Here's how the part is built. I have some questions about the finished solid (model axes, mm). A direction names the side the tool comes from. Coordinates: 2 decimals unless noted, no trailing zeros. Write each loop counter-clockwise with the first axis right and the second up, starting at its lowest first coordinate (ties: lowest second). Pieces come first, ordered by that corner, then holes.
from build123d import *

# Parameters (mm, degrees)
F3_DEPTH = 1.3
F4_R     = 2
F5_DEPTH = 25
F6_SIZE  = 0.3


with BuildPart() as f1:
    # F0 (on Front) → F1 (revolve)
    with BuildSketch(Plane.XZ):
        with BuildLine():
            Line((-3.8, 0), (-3.8, -0.3))
            Line((-3.8, -0.3), (0, -0.3))
            Line((0, -0.3), (0, 1.7))
            Line((0, 1.7), (-2, 1.7))
            ThreePointArc((-2, 1.7), (-3.022003, 0.979179), (-3.8, 0))
        make_face()
    revolve(axis=Axis((0, 0, 0.7), (0, 0, -1)))

    # F2 (on face) → F3 (cut)
    with BuildSketch(Plane.XY.offset(1.7)):
        Polygon((0.721688, 1.25), (-0.721688, 1.25), (-1.443376, 0), (-0.721688, -1.25), (0.721688, -1.25), (1.443376, 0), align=None)
    extrude(amount=-F3_DEPTH, mode=Mode.SUBTRACT)

    # F4 (on face) → F5 (join)
    with BuildSketch(Plane(origin=(0, 0, -0.3), x_dir=(1, 0, 0), z_dir=(0, 0, -1))):
        Circle(F4_R)
    extrude(amount=F5_DEPTH)

    # F6
    f6_edges = [f1.edges().sort_by_distance(p)[0] for p in [
        (-2, 0, -25.3),
    ]]
    chamfer(f6_edges, length=F6_SIZE)


solid = f1.part
1. Thinking about a two-plate mould opening in Y: for faces 1 (the face through (1.088, 0.616, 1.059)), 2 (the face through (0, 0, -25.3)), 3 (the face through (0, 2, -12)), which applies, pulls with the +Y half, pulls with the -Y half, needs draft (parallel to the pull), parting line crosses it, or undercut?
2. On a 3-axis mill with a long thin cutter (end or side, diameter ignored), from which of +Z, -Z, +X, -X, +Y, -Y can I reach the whole of each face in a straight line? I mean faces 4 (the face through (1.08, -0.63, 1.06)), 5 (the face through (-2, -2, -0.3)), 6 (the face through (2.8, 2.57, -0.15)). Say none if no direction works.
3. If I drill on line 1 (Z direction, x = -0.5, y = -0.5); line 2 (X direction, y = 0, z = -20.5), over which ranges is the centre line in solid material (lowest first)?
4. For pin 1 Ø0.6 at (x, z) = (0, 1) entering from -Y; pin 2 Ø3 at (x, y) = (-2.5, 2.5) entering from +Z; pin 3 Ø0.6 at (x, z) = (0, 1) entering from +Y, each with a flat end and sliding along its axis, tell me the tip position at first contact or that it passes through.
5. I want a section at A-A (z = -13.5). List the corners of the cut face in (x, y) for me.
Response values:
1. face 1: undercut
1. face 2: needs draft
1. face 3: parting line crosses it
2. face 4: +Z
2. face 5: -Z
2. face 6: +Z, -Z
3. line 1: z = -25.3 to 0.4
3. line 2: x = -2 to 2
4. pin 1: stops at y = -3.29
4. pin 2: stops at z = 1.68
4. pin 3: stops at y = 3.29
5. outline: circle Ø4 at (0, 0)
